Work out the finished part from the listing and answer in its coordinate system (mm). A direction names the side the tool comes from. Coordinates: 2 decimals unless noted, no trailing zeros. Write each loop counter-clockwise with the first axis right and the second up, starting at its lowest first coordinate (ties: lowest second). Pieces come first, ordered by that corner, then holes. Notation, with made-up numbers: M 24.25,-31 L 78.25,-31 A25 ccw 78.25,-1 Z; hole C -40,52.25 d11. An arc over 180 degrees is marked long. Use CSV: the item, a comma, the result in double quotes.
from build123d import *

# Parameters (mm, degrees)
SKETCH_1_R          = 1.6
SKETCH_1_R_2        = 6.3
SKETCH_1_R_3        = 7.1
EXTRUDE_1_DEPTH     = 5
SKETCH_1_3_R        = 7.1
SKETCH_1_3_R_2      = 2.1
EXTRUDE_2_DEPTH     = 3
FILLET_1_R          = 1
FILLET_2_R          = 1
FILLET_3_R          = 1
FILLET_4_R          = 1
SKETCH_2_R          = 3
CUT_EXTRUDE_1_DEPTH = 1


with BuildPart() as part:
    # Sketch 1 → Extrude 1 (new body)
    with BuildSketch(Plane(origin=(0, 0, 0), x_dir=(1, 0, 0), z_dir=(0, 1, 0))):
        with BuildLine():
            Line((1.305, -14.441155598), (50.9, -9.959417654))
            ThreePointArc((50.9, -9.959417654), (60, 0), (50.9, 9.959417654))
            Line((50.9, 9.959417654), (1.305, 14.441155598))
            ThreePointArc((1.305, 14.441155598), (-14.5, 0), (1.305, -14.441155598))
        make_face()
        with Locations(Location((-10, 0, 0), (0, 0, 270))):
            Circle(SKETCH_1_R, mode=Mode.SUBTRACT)
        with Locations(Location((0, 10, 0), (0, 0, 270))):
            Circle(SKETCH_1_R, mode=Mode.SUBTRACT)
        with Locations(Location((10, 0, 0), (0, 0, 270))):
            Circle(SKETCH_1_R, mode=Mode.SUBTRACT)
        with Locations(Location((0, -10, 0), (0, 0, 270))):
            Circle(SKETCH_1_R, mode=Mode.SUBTRACT)
        with Locations(Location((0, 0, 0), (0, 0, 270))):
            Circle(SKETCH_1_R_2, mode=Mode.SUBTRACT)
        with Locations(Location((50, 0, 0), (0, 0, 270))):
            Circle(SKETCH_1_R_3, mode=Mode.SUBTRACT)
        Polygon((17.540160593, 7.953663379), (37.900667884, 6.113750926), (29.663119838, 2.212910976), align=None, mode=Mode.SUBTRACT)
        Polygon((17.540160593, -7.953663379), (37.900667884, -6.113750926), (29.663119838, -2.212910976), align=None, mode=Mode.SUBTRACT)
        with BuildLine():
            Line((13.42623574, 5.475965106), (24.990033856, 0))
            Line((24.990033856, 0), (13.42623574, -5.475965106))
            ThreePointArc((13.42623574, -5.475965106), (14.5, 0), (13.42623574, 5.475965106))
        make_face(mode=Mode.SUBTRACT)
        with BuildLine():
            Line((34.33620582, 0), (40.424641065, -2.88314087))
            ThreePointArc((40.424641065, -2.88314087), (40, 0), (40.424641065, 2.88314087))
            Line((40.424641065, 2.88314087), (34.33620582, 0))
        make_face(mode=Mode.SUBTRACT)
    extrude(amount=EXTRUDE_1_DEPTH)

    # Sketch 1_3 → Extrude 2 (add)
    with BuildSketch(Plane(origin=(0, 0, 0), x_dir=(1, 0, 0), z_dir=(0, 1, 0))):
        with Locations(Location((50, 0, 0), (0, 0, 270))):
            Circle(SKETCH_1_3_R)
        with Locations(Location((50, 0, 0), (0, 0, 270))):
            Circle(SKETCH_1_3_R_2, mode=Mode.SUBTRACT)
    extrude(amount=EXTRUDE_2_DEPTH)

    # Fillet 1
    fillet_1_edges = [part.edges().sort_by_distance(p)[0] for p in [
        (34.33620582, 2.5, 0),
        (40.424641065, 2.5, 2.88314087),
        (40.424641065, 2.5, -2.88314087),
    ]]
    fillet(fillet_1_edges, radius=FILLET_1_R)

    # Fillet 2
    fillet_2_edges = [part.edges().sort_by_distance(p)[0] for p in [
        (17.540160593, 2.5, 7.953663379),
        (37.900667884, 2.5, 6.113750926),
        (29.663119838, 2.5, 2.212910976),
    ]]
    fillet(fillet_2_edges, radius=FILLET_2_R)

    # Fillet 3
    fillet_3_edges = [part.edges().sort_by_distance(p)[0] for p in [
        (37.900667884, 2.5, -6.113750926),
        (17.540160593, 2.5, -7.953663379),
        (29.663119838, 2.5, -2.212910976),
    ]]
    fillet(fillet_3_edges, radius=FILLET_3_R)

    # Fillet 4
    fillet_4_edges = [part.edges().sort_by_distance(p)[0] for p in [
        (24.990033856, 2.5, 0),
        (13.42623574, 2.5, -5.475965106),
        (13.42623574, 2.5, 5.475965106),
    ]]
    fillet(fillet_4_edges, radius=FILLET_4_R)

    # Sketch 2 → Cut-Extrude 1 (cut)
    with BuildSketch(Plane(origin=(0, 0, 0), x_dir=(1, 0, 0), z_dir=(0, 1, 0))):
        with Locations(Location((0, -10, 0), (0, 0, 270))):
            Circle(SKETCH_2_R)
        with Locations(Location((-10, 0, 0), (0, 0, 270))):
            Circle(SKETCH_2_R)
        with Locations(Location((0, 10, 0), (0, 0, 270))):
            Circle(SKETCH_2_R)
        with Locations(Location((10, 0, 0), (0, 0, 270))):
            Circle(SKETCH_2_R)
    extrude(amount=CUT_EXTRUDE_1_DEPTH, mode=Mode.SUBTRACT)


solid = part.part
Item 1: For a pull along Z with two mould halves and no side action, classify faces 4 (the face through (37.42, 2.46, 1.46)), 5 (the face through (60, 2, 0)), 6 (the face through (26.45, 2.46, -12.17)) as released by +Z, released by -Z, zero draft, split by the parting line, or undercut.
Answer:
face 4,"undercut"
face 5,"split by the parting line"
face 6,"released by -Z"
Item 2: The part is cut by section C-C (x = 19). Write down the section's boundary in (y, z), then the cut area to 3 significant figures.
Answer:
outline,"M 0,-12.84 L 5,-12.84 L 5,-2.84 L 0,-2.84 Z; M 0,2.84 L 5,2.84 L 5,12.84 L 0,12.84 Z"
area,"100 mm2"
Item 3: A tool of negligible diameter and unlimited length cuts with its end or side. For faces 1 (the face through (-1.3, 1, 11.3)), 2 (the face through (35.673, 2.535, 0.016)), 3 (the face through (48.5, 3, -1.7)), from which of +Z, -Z, +X, -X, +Y, -Y can it reach the whole face along a straight path? Write none if from no direction.
Answer:
face 1,"-Y"
face 2,"+Y, -Y"
face 3,"+Y"
Item 4: Consider probe 1 along X at (y, z) = (1.6, -4.25); probe 2 along Y at (x, z) = (47.5, -1); probe 3 along Z at (x, y) = (23, 3.85). Determine where each line is inside the solid, lowest interval first.
Answer:
probe 1,"x = -13.86 to -4.65, 4.65 to 14.33, 16.02 to 25.36, 33.96 to 59.05"
probe 2,"y = 0 to 3"
probe 3,"z = -12.48 to -7.45, -5.37 to -0.94, 0.94 to 5.37, 7.45 to 12.48"
Item 5: The part is cut by section A-A (x = 0). Write down the section's boundary in (y, z), then the cut area to 3 significant figures.
Answer:
outline,"M 0,-14.5 L 5,-14.5 L 5,-11.6 L 1,-11.6 L 1,-13 L 0,-13 Z; M 0,-7 L 1,-7 L 1,-8.4 L 5,-8.4 L 5,-6.3 L 0,-6.3 Z; M 0,6.3 L 5,6.3 L 5,8.4 L 1,8.4 L 1,7 L 0,7 Z; M 0,13 L 1,13 L 1,11.6 L 5,11.6 L 5,14.5 L 0,14.5 Z"
area,"44.4 mm2"
Item 6: The part is cut by section D-D (z = -10.75). Write down the section's boundary in (x, y).
Answer:
outline,"M -9.73,0 L -2.9,0 L -2.9,1 L -1.41,1 L -1.41,5 L -9.73,5 Z; M 1.41,1 L 2.9,1 L 2.9,0 L 42.15,0 L 42.15,5 L 1.41,5 Z"
Item 7: Given pin 1 (1.8 mm diameter, centred on x = 11, z = 0.5, fed in from -Y); pin 2 (4.5 mm diameter, centred on x = 51.5, z = -2, fed in from +Y); pin 3 (1 mm diameter, centred on x = 51.5, y = 3, fed in from -Z), each flat-ended and moving along its own axis, determine where each tip first touches the part or whether it passes through.
Answer:
pin 1,"stops at y = 1"
pin 2,"stops at y = 3"
pin 3,"stops at z = -9.95"
Item 8: The part is cut by section B-B (z = 0). Count the separate pieces of the cut face and the enclosed holes in it, then the cut area to 3 significant figures.
Answer:
separate pieces,"7"
enclosed holes,"0"
area,"163 mm2"
